```python
from build123d import *

# Parameters (mm, degrees)
SKETCH1_W           = 60
SKETCH1_H           = 40
SKETCH1_W_2         = 25
SKETCH1_H_2         = 15
SKETCH1_R           = 1.59
SKETCH1_R_2         = 4.5
BOSS_EXTRUDE1_DEPTH = 6.35


with BuildPart() as part:
    # Sketch1 → Boss-Extrude1 (new body)
    # profile 1 of 2: a face of its own
    with BuildSketch(Plane.XY):
        with Locations((30, -20)):
            Rectangle(SKETCH1_W, SKETCH1_H)
        with Locations((30, -30)):
            Rectangle(SKETCH1_W_2, SKETCH1_H_2, mode=Mode.SUBTRACT)
    # profile 2 of 2: a face of its own
    with BuildSketch(Plane.XY):
        with Locations((30, -30)):
            Rectangle(SKETCH1_W_2, SKETCH1_H_2)
        with Locations((39, -30)):
            Circle(SKETCH1_R, mode=Mode.SUBTRACT)
        with Locations((21, -30)):
            Circle(SKETCH1_R, mode=Mode.SUBTRACT)
        with Locations((30, -30)):
            Circle(SKETCH1_R_2, mode=Mode.SUBTRACT)
    extrude(amount=BOSS_EXTRUDE1_DEPTH)


solid = part.part
```
The listing builds one solid part. Answer for the finished solid, in the listing's coordinates (mm). Coordinates: 2 decimals unless noted, no trailing zeros. Write each loop counter-clockwise with the first axis right and the second up, starting at its lowest first coordinate (ties: lowest second). Pieces come first, ordered by that corner, then holes. Notation, with made-up numbers: M 0.25,81 L 59.25,81 A14 cw 59.25,106 Z; hole C -35,39.25 d1. An arc over 180 degrees is marked long. Use a Markdown table: item, result. Add a question column.
1. Section B-B (z = 3) is taken. Give the vertices of the cut face in (x, y), plus the area to 3 significant figures.
2. Section A-A (x = 21) is taken. Give the vertices of the cut face in (y, z), plus the area to 3 significant figures.
3. Given P1, Ø7, axis at x = 30, y = -30, coming from the -Z side, flat-ended and moving along its own axis, determine where the tip first touches the part or whether it passes through.
4. Section C-C (y = -30) is taken. Give the vertices of the cut face in (x, z).
5. Section D-D (x = 30) is taken. Give the vertices of the cut face in (y, z), plus the area to 3 significant figures.
6. Straight lines are drawn through the part: line 1 along Y through (x, z) = (21, 3.5); line 2 along X through (y, z) = (-29, 1.5); line 3 along Y through (x, z) = (38.5, 3). For each, find the intervals that lie inside material, in ascending order. Write a range as [from, to].
7. For a pull along X with two mould halves and no side action, classify faces 1 (the flat face through (0, -20, 3)), 2 (the flat face through (30, -20, 6.35)), 3 (the flat face through (60, -20, 3)), 4 (the cylindrical face through (32.08, -33.99, 3.13)) as +X half, -X half, draft (parallel to the pull), parting line (faces both ways), or undercut.
Data:
| question | item | result |
|---|---|---|
| 1 | outline | M 0,-40 L 60,-40 L 60,0 L 0,0 Z; hole C 21,-30 d3.18; hole C 30,-30 d9; hole C 39,-30 d3.18 |
| 1 | area | 2,320 mm2 |
| 2 | outline | M -40,0 L -31.59,0 L -31.59,6.35 L -40,6.35 Z; M -28.41,0 L 0,0 L 0,6.35 L -28.41,6.35 Z |
| 2 | area | 234 mm2 |
| 3 | P1 | passes through |
| 4 | outline | M 0,0 L 19.41,0 L 19.41,6.35 L 0,6.35 Z; M 22.59,0 L 25.5,0 L 25.5,6.35 L 22.59,6.35 Z; M 34.5,0 L 37.41,0 L 37.41,6.35 L 34.5,6.35 Z; M 40.59,0 L 60,0 L 60,6.35 L 40.59,6.35 Z |
| 5 | outline | M -40,0 L -34.5,0 L -34.5,6.35 L -40,6.35 Z; M -25.5,0 L 0,0 L 0,6.35 L -25.5,6.35 Z |
| 5 | area | 197 mm2 |
| 6 | line 1 | y = [-40, -31.59], [-28.41, 0] |
| 6 | line 2 | x = [0, 19.76], [22.24, 25.61], [34.39, 37.76], [40.24, 60] |
| 6 | line 3 | y = [-40, -31.51], [-28.49, 0] |
| 7 | face 1 | -X half |
| 7 | face 2 | draft |
| 7 | face 3 | +X half |
| 7 | face 4 | undercut |
